Can you work these out from the model? Positions are in its coordinate system, mm. Round coordinates to 2 decimals unless told otherwise and drop trailing zeros. Order: outer loops, then holes, each group sorted by start corner. A loop starts at its lowest first (then second) coordinate and runs counter-clockwise, first axis right, second up. Notation, with made-up numbers: (57, -6) -> (68, -6) arc R22 ccw to (68, 29) -> close; hole circle Ø9 at (-38.75, 16.25). An arc over 180 degrees is marked (long way). Use a Markdown table: item, result. Add a question column.
Q1. If we section it at B-B on x = 0: List the corners of the cut face in (y, z) for me (3 decimals), plus the area to 3 significant figures.
Q2. If we section it at A-A on z = 0: List the corners of the cut face in (x, y) for me.
Q3. I need wall thicknesses on line 1 along X through (y, z) = (2.15, 0). Which ranges of the line are inside material? Lowest first, please. Write a range as [from, to].
Q4. If we section it at C-C on y = 1.6: List the corners of the cut face in (x, z) for me, plus the area to 3 significant figures.
Q5. If we section it at D-D on x = 60: List the corners of the cut face in (y, z) for me (3 decimals), plus the area to 3 significant figures.
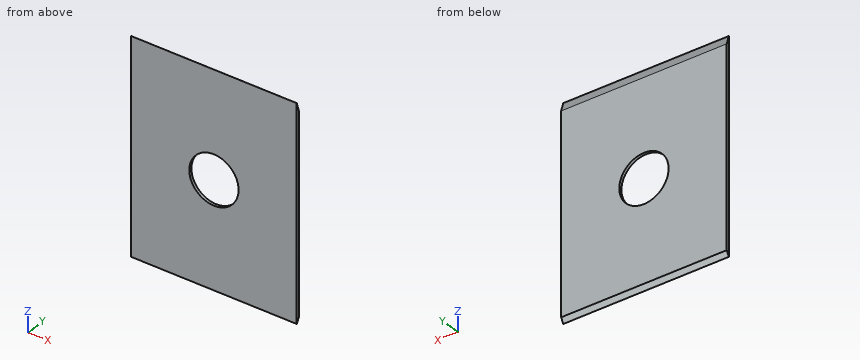
```python
from build123d import *

# Parameters (mm, degrees)
ESQUISSE1_W             = 174.68
ESQUISSE1_H             = 223.37
ESQUISSE1_R             = 26
BOSS_EXTRU_1_DEPTH      = 3
ENL_V_MAT_EXTRU_1_DEPTH = 190


with BuildPart() as part:
    # Esquisse1 → Boss.-Extru.1 (new body)
    with BuildSketch(Plane(origin=(0, 0, 0), x_dir=(1, 0, 0), z_dir=(0, 1, 0))):
        Rectangle(ESQUISSE1_W, ESQUISSE1_H)
        Circle(ESQUISSE1_R, mode=Mode.SUBTRACT)
    extrude(amount=BOSS_EXTRU_1_DEPTH)

    # Esquisse2 → Enlèv. mat.-Extru.1 (cut)
    with BuildSketch(Plane.ZY.offset(87.34)):
        Polygon((-111.685, 0), (-106.491722689, 3), (-111.685, 3), align=None)
        Polygon((102.233000386, 3), (111.685, 0.028240342), (111.685, 3), align=None)
    extrude(amount=-ENL_V_MAT_EXTRU_1_DEPTH, mode=Mode.SUBTRACT)


solid = part.part
```
Answer below:
| question | item | result |
|---|---|---|
| 1 | outline | (0, -111.685) -> (3, -106.492) -> (3, -26) -> (0, -26) -> close; (0, 26) -> (3, 26) -> (3, 102.233) -> (0.028, 111.685) -> (0, 111.685) -> close |
| 1 | area | 492 mm² |
| 2 | outline | (-87.34, 0) -> (-26, 0) -> (-26, 3) -> (-87.34, 3) -> close; (26, 0) -> (87.34, 0) -> (87.34, 3) -> (26, 3) -> close |
| 3 | line 1 | [-87.34, -26], [26, 87.34] |
| 4 | outline | (-87.34, -108.92) -> (87.34, -108.92) -> (87.34, 106.69) -> (-87.34, 106.69) -> close; hole circle Ø52 at (0, 0) |
| 4 | area | 35,500 mm² |
| 5 | outline | (0, -111.685) -> (3, -106.492) -> (3, 102.233) -> (0.028, 111.685) -> (0, 111.685) -> close |
| 5 | area | 648 mm² |
